```python
from build123d import *

# Parameters (mm, degrees)
SKETCH4_R           = 0.75
CUT_EXTRUDE2_DEPTH  = 4
BOSS_EXTRUDE2_DEPTH = 1


with BuildPart() as part:
    # Sketch1 → Revolve1 (revolve)
    with BuildSketch(Plane(origin=(0, 0, 0), x_dir=(0, 0, -1), z_dir=(1, 0, 0))):
        with BuildLine():
            ThreePointArc((-3, 4), (-2.121320344, 1.878679656), (0, 1))
            Line((0, 1), (0, 0))
            Line((0, 0), (0, -9.5))
            Line((0, -9.5), (0, -15.1))
            ThreePointArc((0, -15.1), (-2.753447859, -12.808453427), (-1, -9.684660634))
            Line((-1, -9.684660634), (-1, 0.127016654))
            ThreePointArc((-1, 0.127016654), (-2.123180734, 0.609999474), (-3.048002331, 1.409694653))
            Line((-3.048002331, 1.409694653), (-16, 3))
            Line((-16, 3), (-16, 4))
            Line((-16, 4), (-4, 4))
            Line((-4, 4), (-3, 4))
        make_face()
    revolve(axis=Axis((0, 10.634252877, 0), (0, 1, 0)))

    # Sketch4 → Cut-Extrude2 (cut)
    with BuildSketch(Plane(origin=(0, 4, 0), x_dir=(1, 0, 0), z_dir=(0, 1, 0))):
        with BuildLine():
            Line((-1.08219807, 4.881480036), (-3.030154595, 13.6681441))
            ThreePointArc((-3.030154595, 13.6681441), (-9.899494937, 9.899494937), (-13.6681441, 3.030154595))
            Line((-13.6681441, 3.030154595), (-4.881480036, 1.08219807))
            ThreePointArc((-4.881480036, 1.08219807), (-3.535533906, 3.535533906), (-1.08219807, 4.881480036))
        make_face()
        with BuildLine():
            Line((-4.881480036, -1.08219807), (-13.6681441, -3.030154595))
            ThreePointArc((-13.6681441, -3.030154595), (-9.899494937, -9.899494937), (-3.030154595, -13.6681441))
            Line((-3.030154595, -13.6681441), (-1.08219807, -4.881480036))
            ThreePointArc((-1.08219807, -4.881480036), (-3.535533906, -3.535533906), (-4.881480036, -1.08219807))
        make_face()
        with BuildLine():
            ThreePointArc((3.030154595, -13.6681441), (9.899494937, -9.899494937), (13.6681441, -3.030154595))
            Line((13.6681441, -3.030154595), (4.881480036, -1.08219807))
            ThreePointArc((4.881480036, -1.08219807), (3.535533906, -3.535533906), (1.08219807, -4.881480036))
            Line((1.08219807, -4.881480036), (3.030154595, -13.6681441))
        make_face()
        with BuildLine():
            ThreePointArc((13.6681441, 3.030154595), (9.899494937, 9.899494937), (3.030154595, 13.6681441))
            Line((3.030154595, 13.6681441), (1.08219807, 4.881480036))
            ThreePointArc((1.08219807, 4.881480036), (3.535533906, 3.535533906), (4.881480036, 1.08219807))
            Line((4.881480036, 1.08219807), (13.6681441, 3.030154595))
        make_face()
        with Locations(Location((-14, 0, 0), (0, 0, 134.876670286))):
            Circle(SKETCH4_R)
        with Locations(Location((-10, 0, 0), (0, 0, 43.63623207))):
            Circle(SKETCH4_R)
        with Locations(Location((0, 10, 0), (0, 0, 270))):
            Circle(SKETCH4_R)
        with Locations(Location((0, 14, 0), (0, 0, 270))):
            Circle(SKETCH4_R)
        with Locations(Location((0, -10, 0), (0, 0, 90))):
            Circle(SKETCH4_R)
        with Locations(Location((0, -14, 0), (0, 0, 270.000000015))):
            Circle(SKETCH4_R)
        with Locations(Location((10, 0, 0), (0, 0, 270))):
            Circle(SKETCH4_R)
        with Locations(Location((14, 0, 0), (0, 0, 270))):
            Circle(SKETCH4_R)
    extrude(amount=-CUT_EXTRUDE2_DEPTH, mode=Mode.SUBTRACT)

    # Sketch5 → Boss-Extrude2 (add)
    with BuildSketch(Plane(origin=(0, 4, 0), x_dir=(1, 0, 0), z_dir=(0, 1, 0))):
        with BuildLine():
            ThreePointArc((-11.998696572, 10.584483009), (-11.313708499, 11.313708499), (-10.584483009, 11.998696572))
            Line((-10.584483009, 11.998696572), (-16, 16))
            Line((-16, 16), (-11.998696572, 10.584483009))
        make_face()
        with BuildLine():
            Line((16, 16), (10.584483009, 11.998696572))
            ThreePointArc((10.584483009, 11.998696572), (11.313708499, 11.313708499), (11.998696572, 10.584483009))
            Line((11.998696572, 10.584483009), (16, 16))
        make_face()
        with BuildLine():
            ThreePointArc((11.998696572, -10.584483009), (11.313708499, -11.313708499), (10.584483009, -11.998696572))
            Line((10.584483009, -11.998696572), (16, -16))
            Line((16, -16), (11.998696572, -10.584483009))
        make_face()
        with BuildLine():
            ThreePointArc((-10.584483009, -11.998696572), (-11.313708499, -11.313708499), (-11.998696572, -10.584483009))
            Line((-11.998696572, -10.584483009), (-16, -16))
            Line((-16, -16), (-10.584483009, -11.998696572))
        make_face()
    extrude(amount=-BOSS_EXTRUDE2_DEPTH)


solid = part.part
```
Work out the finished part from the listing and answer in its coordinate system (mm). A direction names the side the tool comes from. Round coordinates to 2 decimals unless told otherwise and drop trailing zeros. Write each loop counter-clockwise with the first axis right and the second up, starting at its lowest first coordinate (ties: lowest second). Pieces come first, ordered by that corner, then holes. Notation, with made-up numbers: (-23.5, 69) -> (26.5, 69) arc R20 ccw to (26.5, 77) -> close; hole circle Ø11 at (68, -10). An arc over 180 degrees is marked (long way). Write each question's results on one line, items separated by ' | '.
Q1. Section A-A, the plane x = 0 is taken. Write down the section's boundary in (y, z).
Data:
outline: (-9.68, -1) -> (0.13, -1) arc R4 ccw to (1.41, -3.05) -> (2.17, -9.25) -> (4, -9.25) -> (4, -3) arc R3 cw to (4, 3) -> (4, 9.25) -> (2.17, 9.25) -> (1.41, 3.05) arc R4 ccw to (0.13, 1) -> (-9.68, 1) arc R2.8 ccw (long way) to start; (2.36, -10.75) -> (2.66, -13.25) -> (4, -13.25) -> (4, -10.75) -> close; (2.36, 10.75) -> (4, 10.75) -> (4, 13.25) -> (2.66, 13.25) -> close; (2.85, -14.75) -> (3, -16) -> (4, -16) -> (4, -14.75) -> close; (2.85, 14.75) -> (4, 14.75) -> (4, 16) -> (3, 16) -> close
Q2. Which of the six approach directions +Z, -Z, +X, -X, +Y, -Y give full straight-line access (tool end or side, diameter ignored) to faces 5 (the flat face through (13.33, 3.507, -14.027)), 6 (the flat face through (-14.027, 3.507, -13.33)), 7 (the cylindrical face through (16, 3.5, 0.2)), 8 (the flat face through (13, 3, 13)), 9 (the cylindrical face through (-10, 3.4, 9.8))?
Data:
face 5: -Z, +Y, -Y | face 6: -X, +Y, -Y | face 7: +X, +Y, -Y | face 8: +Z, +X, -Y | face 9: +Y, -Y
Q3. Straight lines are drawn through the part: line 1 along X through (y, z) = (3.1, 14); line 2 along Z through (x, y) = (-0.5, 3.25); line 3 along X through (y, z) = (3.3, 10). For each, find the intervals that lie inside material, in ascending order. Write a range as [from, to].
Data:
line 1: [-14.52, -13.29], [-7.75, -0.75], [0.75, 7.75], [13.29, 14.52] | line 2: [-15.99, -14.56], [-13.44, -10.56], [-9.44, -2.86], [2.86, 9.44], [10.56, 13.44], [14.56, 15.99] | line 3: [-12.49, -9.8], [-2.22, -0.75], [0.75, 2.22], [9.8, 12.49]
Q4. Determine the mould class of faces 1 (the flat face through (-2.04, 3.1, -9.21)), 2 (the cylindrical face through (0.2, 3.5, -16)), 3 (the cylindrical face through (0.03, 3.34, 13.25)), 4 (the conical face through (2.61, 1.51, -2.84)) for opening direction Z: released by +Z, released by -Z, zero draft, split by the parting line, or undercut.
Data:
face 1: undercut | face 2: released by -Z | face 3: undercut | face 4: split by the parting line
Q5. Section B-B, the plane z = 12.5 is taken. Give the number of separate pieces and of enclosed holes in the cut face, then the cut area to 3 significant figures.
Data:
separate pieces: 5 | enclosed holes: 0 | area: 20.5 mm^2
Q6. Section C-C, the plane y = -2.25 is taken. Write down the section's boundary in (x, z).
Data:
outline: circle Ø2 at (0, 0)
Q7. Flat-ended cylindrical pins translate along their axes: P1, Ø6, axis at x = 12.5, z = -13, coming from the -Y side; P2, Ø6, axis at x = 14, z = 14.5, coming from the -Y side; P3, Ø5, axis at x = -0.5, y = -8.5, coming from the +Z side; P4, Ø0.9, axis at x = 14, z = 0, coming from the +Y side. Find the tip coordinate at first contact, or state that the pin passes through.
Data:
P1: y = 2.88 | P2: y = 3 | P3: z = 2.46 | P4: through
